Could you check a few things on this model? Use its own coordinates, in mm. A direction names the side the tool comes from. Round coordinates to 2 decimals unless told otherwise and drop trailing zeros. Loops run counter-clockwise (first coordinate to the right, second up) from the corner with the lowest first, then second, coordinate; pieces in that order, holes last. Notation, with made-up numbers: (48.25, -27.75) - (79.25, -27.75) arc R25 cw to (79.25, 4.25) - close; hole circle Ø3 at (-34.5, 38.5). An arc over 180 degrees is marked (long way). Use one line per item in the form item = value.
```python
from build123d import *

# Parameters (mm, degrees)
SKETCH2_R           = 26.5
BOSS_EXTRUDE1_DEPTH = 200
SKETCH3_R           = 5
BOSS_EXTRUDE2_DEPTH = 35
SKETCH4_R           = 10.271360286
BOSS_EXTRUDE3_DEPTH = 15
SKETCH5_R           = 19.288260132
BOSS_EXTRUDE4_DEPTH = 5


with BuildPart() as part:
    # Sketch2 → Boss-Extrude1 (new body)
    with BuildSketch(Plane.XY):
        with Locations((29.69848481, 29.69848481)):
            Circle(SKETCH2_R)
    extrude(amount=BOSS_EXTRUDE1_DEPTH)

    # Sketch3 → Boss-Extrude2 (add)
    with BuildSketch(Plane.XY.offset(200)):
        with Locations((29.69848481, 29.69848481)):
            Circle(SKETCH3_R)
    extrude(amount=BOSS_EXTRUDE2_DEPTH)

    # Sketch4 → Boss-Extrude3 (add)
    with BuildSketch(Plane(origin=(0, 0, 0), x_dir=(-1, 0, 0), z_dir=(0, 0, -1))):
        with Locations((-29.69848481, 29.69848481)):
            Circle(SKETCH4_R)
    extrude(amount=BOSS_EXTRUDE3_DEPTH)

    # Sketch5 → Boss-Extrude4 (add)
    with BuildSketch(Plane(origin=(0, 0, -15), x_dir=(-1, 0, 0), z_dir=(0, 0, -1))):
        with Locations((-29.69848481, 29.69848481)):
            Circle(SKETCH5_R)
    extrude(amount=BOSS_EXTRUDE4_DEPTH)


solid = part.part
```
1. Please list where these lines run through material, in increasing order: line 1 along Z through (x, y) = (40, 44.5); line 2 along Z through (x, y) = (10, 16.5); line 3 along X through (y, z) = (29.5, 201).
Solution:
line_1 = -20 to -15, 0 to 200
line_2 = 0 to 200
line_3 = 24.7 to 34.69
2. On a 3-axis mill with a long thin cutter (end or side, diameter ignored), from which of +Z, -Z, +X, -X, +Y, -Y can I reach the whole of each face in a straight line? I mean faces 4 (the face through (19.329, 45.962, -17.465)), 5 (the face through (30, 30, 235)), 6 (the face through (41, 30, 0)). Say none if no direction works.
Solution:
face_4 = -Z
face_5 = +Z, +X, -X, +Y, -Y
face_6 = none
3. If we section it at A-A, the plane y = 15: Write out the boundary of the cut face in (x, z).
Solution:
outline = (7.65, 0) - (51.75, 0) - (51.75, 200) - (7.65, 200) - close; (17.21, -20) - (42.19, -20) - (42.19, -15) - (17.21, -15) - close
4. We'd pull the mould along Z, two halves only. Please class faces 1 (the face through (39.96, 30.15, -7.4)), 2 (the face through (32.006, 25.263, 217.255)), 3 (the face through (35, 30, 200)): +Z half, -Z half, draft (parallel to the pull), parting line (faces both ways), or undercut.
Solution:
face_1 = undercut
face_2 = draft
face_3 = +Z half
5. For P1, Ø3, axis at y = 20.5, z = 31, coming from the -X side; P2, Ø1, axis at x = 32.5, z = 43, coming from the -Y side; P3, Ø10, axis at x = 48.5, z = 43, coming from the +Y side; P4, Ø1, axis at x = 50, y = 9.5, coming from the +Z side, each with a flat end and sliding along its axis, tell me the tip position at first contact or that it passes through.
Solution:
P1 = 4.34
P2 = 3.3
P3 = 52.32
P4 = through
6. If we section it at C-C, the plane x = 32.5: Write out the boundary of the cut face in (y, z), plus the area to 3 significant figures.
Solution:
outline = (3.35, 0) - (19.82, 0) - (19.82, -15) - (10.61, -15) - (10.61, -20) - (48.78, -20) - (48.78, -15) - (39.58, -15) - (39.58, 0) - (56.05, 0) - (56.05, 200) - (33.84, 200) - (33.84, 235) - (25.56, 235) - (25.56, 200) - (3.35, 200) - close
area = 11,300 mm^2
7. If we section it at B-B, the plane x = 45: Write out the boundary of the cut face in (y, z), plus the area to 3 significant figures.
Solution:
outline = (8.06, 0) - (51.33, 0) - (51.33, 200) - (8.06, 200) - close; (17.96, -20) - (41.44, -20) - (41.44, -15) - (17.96, -15) - close
area = 8,770 mm^2
8. If we section it at D-D, the plane z = 56.5: Write out the boundary of the cut face in (x, y), plus the area to 3 significant figures.
Solution:
outline = circle Ø53 at (29.7, 29.7)
area = 2,210 mm^2
